```python
from build123d import *

# Parameters (mm, degrees)
F0_R     = 1
F0_W     = 6
F0_H     = 60
F1_DEPTH = 5


with BuildPart() as f1:
    # F0 (on Top) → F1 (new body)
    with BuildSketch(Plane.XY):
        Polygon((-117.94585, -363), (18.319213, -363), (18.319213, 363), (-117.94585, 363), (-308.786243, 224.346338), (-381.680787, 0), (-308.786243, -224.346338), align=None)
        with Locations((-297.727783, -228.672576)):
            Circle(F0_R, mode=Mode.SUBTRACT)
        with Locations((-309.483488, -212.492236)):
            Circle(F0_R, mode=Mode.SUBTRACT)
        with Locations((-314.118743, -198.226388)):
            Circle(F0_R, mode=Mode.SUBTRACT)
        with Locations((-285.592528, -237.489355)):
            Circle(F0_R, mode=Mode.SUBTRACT)
        with Locations((-125.477599, -353.81966)):
            Circle(F0_R, mode=Mode.SUBTRACT)
        with Locations((-137.612854, -345.002881)):
            Circle(F0_R, mode=Mode.SUBTRACT)
        with Locations((-106.456468, -360)):
            Circle(F0_R, mode=Mode.SUBTRACT)
        with Locations((-91.456468, -360)):
            Circle(F0_R, mode=Mode.SUBTRACT)
        with Locations((-370.641949, -24.265848)):
            Circle(F0_R, mode=Mode.SUBTRACT)
        with Locations((-375.277204, -10)):
            Circle(F0_R, mode=Mode.SUBTRACT)
        with Locations((-375.277204, 10)):
            Circle(F0_R, mode=Mode.SUBTRACT)
        with Locations((-370.641949, 24.265848)):
            Circle(F0_R, mode=Mode.SUBTRACT)
        with Locations((-314.118743, 198.226388)):
            Circle(F0_R, mode=Mode.SUBTRACT)
        with Locations((-309.483488, 212.492236)):
            Circle(F0_R, mode=Mode.SUBTRACT)
        with Locations((-297.727783, 228.672576)):
            Circle(F0_R, mode=Mode.SUBTRACT)
        with Locations((-285.592528, 237.489355)):
            Circle(F0_R, mode=Mode.SUBTRACT)
        with Locations((-137.612854, 345.002881)):
            Circle(F0_R, mode=Mode.SUBTRACT)
        with Locations((-125.477599, 353.81966)):
            Circle(F0_R, mode=Mode.SUBTRACT)
        with Locations((-106.456468, 360)):
            Circle(F0_R, mode=Mode.SUBTRACT)
        with Locations((-91.456468, 360)):
            Circle(F0_R, mode=Mode.SUBTRACT)
        Rectangle(F0_W, F0_H, mode=Mode.SUBTRACT)
    extrude(amount=F1_DEPTH)


solid = f1.part
```
Design review of the part built by this model. Coordinates are the model's own, in mm. Coordinates: 2 decimals unless noted, no trailing zeros. Order: outer loops, then holes, each group sorted by start corner. A loop starts at its lowest first (then second) coordinate and runs counter-clockwise, first axis right, second up.
1) Take a section at A-A, the plane z = 2.45. State how many separate pieces and enclosed holes the cut face has, and give its area (3 significant figures).
2) Clearance check with flat-ended pins moving along their axes: pin 1 (1.5 mm diameter, centred on y = -246, z = 3.5, fed in from -X); pin 2 (2.5 mm diameter, centred on x = -370.64, y = -24.27, fed in from +Z); pin 3 (1 mm diameter, centred on x = -280, z = 2, fed in from +Y); pin 4 (3 mm diameter, centred on y = -166.5, z = 2.5, fed in from -X). State where each tip first meets the part, or that it passes through.
3) Take a section at B-B, the plane x = -195.5. Give the boundary of the cut face in (y, z), and give its area (3 significant figures).
4) Take a section at C-C, the plane y = -66. Give the boundary of the cut face in (x, z), and give its area (3 significant figures).
5) Wall thickness on line 1 along X through (y, z) = (-360, 3.45) (3 decimals); line 2 along X through (y, z) = (22, 1.6); line 3 along Y through (x, z) = (-230, 4): over which ranges is each line inside the solid? List them lowest first.
Returned:
1. separate pieces: 1
1. enclosed holes: 21
1. area: 227,000 mm2
2. pin 1: stops at x = -280.01
2. pin 2: stops at z = 5
2. pin 3: stops at y = 245.62
2. pin 4: stops at x = -328.07
3. outline: (-306.65, 0) - (306.65, 0) - (306.65, 5) - (-306.65, 5) - close
3. area: 3,070 mm2
4. outline: (-360.24, 0) - (18.32, 0) - (18.32, 5) - (-360.24, 5) - close
4. area: 1,890 mm2
5. line 1: x = -122.075 to -107.456, -105.456 to -92.456, -90.456 to 18.319
5. line 2: x = -374.53 to -3, 3 to 18.32
5. line 3: y = -281.59 to 281.59
